Work out the finished part from the listing and answer in its coordinate system (mm). A direction names the side the tool comes from. Give positions to 0.01 mm unless a question says otherwise; leave off trailing zeros. Order: outer loops, then holes, each group sorted by start corner. A loop starts at its lowest first (then second) coordinate and runs counter-clockwise, first axis right, second up. Notation, with made-up numbers: (51.25, 36) - (76.25, 36) arc R27 ccw to (76.25, 61) - close; hole circle Ø10 at (7.5, 67.25). An arc over 180 degrees is marked (long way). Put each result on its own line as item: value.
```python
from build123d import *

# Parameters (mm, degrees)
CROQUIS2_W              = 51
CROQUIS2_H              = 50
SALIENTE_EXTRUIR3_DEPTH = 10
CROQUIS6_W              = 49
CROQUIS6_H              = 9
CORTAR_EXTRUIR4_DEPTH   = 50
CORTAR_EXTRUIR5_REACH   = 38.827
CROQUIS7_R              = 0.25
CORTAR_EXTRUIR7_REACH   = 38.827
CROQUIS10_R             = 0.25
CORTAR_EXTRUIR8_REACH   = 38.827
CROQUIS11_R             = 0.25
CORTAR_EXTRUIR9_REACH   = 38.827
CROQUIS12_R             = 0.25
CORTAR_EXTRUIR10_REACH  = 38.827
CROQUIS13_R             = 0.35


with BuildPart() as part:
    # Croquis2 → Saliente-Extruir3 (new body)
    with BuildSketch(Plane(origin=(0, 0, 0), x_dir=(1, 0, 0), z_dir=(0, 1, 0))):
        Rectangle(CROQUIS2_W, CROQUIS2_H)
    extrude(amount=SALIENTE_EXTRUIR3_DEPTH)

    # Croquis6 → Cortar-Extruir4 (cut)
    with BuildSketch(Plane.XY.offset(25)):
        with Locations((0, 5.5)):
            Rectangle(CROQUIS6_W, CROQUIS6_H)
    extrude(amount=-CORTAR_EXTRUIR4_DEPTH, mode=Mode.SUBTRACT)

    # Croquis7 → Cortar-Extruir5 (cut, up to next)
    with BuildSketch(Plane(origin=(0, 1, 0), x_dir=(1, 0, 0), z_dir=(0, 1, 0)), mode=Mode.PRIVATE) as cortar_extruir5_sk1:
        with Locations(Location((-20, 22.5, 0), (0, 0, 270))):
            Circle(CROQUIS7_R)
    cortar_extruir5_tool1 = extrude(cortar_extruir5_sk1.sketch, amount=-CORTAR_EXTRUIR5_REACH, mode=Mode.PRIVATE) & part.part
    add(cortar_extruir5_tool1.solids().sort_by_distance((-20, 1, -22.5))[0], mode=Mode.SUBTRACT)

    # Croquis10 → Cortar-Extruir7 (cut, up to next)
    with BuildSketch(Plane(origin=(0, 1, 0), x_dir=(1, 0, 0), z_dir=(0, 1, 0)), mode=Mode.PRIVATE) as cortar_extruir7_sk1:
        with Locations(Location((20, 22.5, 0), (0, 0, 270))):
            Circle(CROQUIS10_R)
    cortar_extruir7_tool1 = extrude(cortar_extruir7_sk1.sketch, amount=-CORTAR_EXTRUIR7_REACH, mode=Mode.PRIVATE) & part.part
    add(cortar_extruir7_tool1.solids().sort_by_distance((20, 1, -22.5))[0], mode=Mode.SUBTRACT)

    # Croquis11 → Cortar-Extruir8 (cut, up to next)
    with BuildSketch(Plane(origin=(0, 1, 0), x_dir=(1, 0, 0), z_dir=(0, 1, 0)), mode=Mode.PRIVATE) as cortar_extruir8_sk1:
        with Locations(Location((-20, -22.5, 0), (0, 0, 270))):
            Circle(CROQUIS11_R)
    cortar_extruir8_tool1 = extrude(cortar_extruir8_sk1.sketch, amount=-CORTAR_EXTRUIR8_REACH, mode=Mode.PRIVATE) & part.part
    add(cortar_extruir8_tool1.solids().sort_by_distance((-20, 1, 22.5))[0], mode=Mode.SUBTRACT)

    # Croquis12 → Cortar-Extruir9 (cut, up to next)
    with BuildSketch(Plane(origin=(0, 1, 0), x_dir=(1, 0, 0), z_dir=(0, 1, 0)), mode=Mode.PRIVATE) as cortar_extruir9_sk1:
        with Locations(Location((20, -22.5, 0), (0, 0, 270))):
            Circle(CROQUIS12_R)
    cortar_extruir9_tool1 = extrude(cortar_extruir9_sk1.sketch, amount=-CORTAR_EXTRUIR9_REACH, mode=Mode.PRIVATE) & part.part
    add(cortar_extruir9_tool1.solids().sort_by_distance((20, 1, 22.5))[0], mode=Mode.SUBTRACT)

    # Croquis13 → Cortar-Extruir10 (cut, up to next)
    with BuildSketch(Plane(origin=(0, 1, 0), x_dir=(1, 0, 0), z_dir=(0, 1, 0)), mode=Mode.PRIVATE) as cortar_extruir10_sk1:
        with Locations(Location((1.077350269, -16.5, 0), (0, 0, 270))):
            Circle(CROQUIS13_R)
    cortar_extruir10_tool1 = extrude(cortar_extruir10_sk1.sketch, amount=-CORTAR_EXTRUIR10_REACH, mode=Mode.PRIVATE) & part.part
    add(cortar_extruir10_tool1.solids().sort_by_distance((1.07735, 1, 16.5))[0], mode=Mode.SUBTRACT)


solid = part.part
```
(1) Section C-C, the plane x = -15 is taken. Write down the section's boundary in (y, z).
Geometry check:
outline: (0, -25) - (1, -25) - (1, 25) - (0, 25) - close
(2) Straight lines are drawn through the part: line 1 (Z direction, x = -20, y = 0.35); line 2 (X direction, y = 0.4, z = -22.5); line 3 (X direction, y = 9.75, z = 18). For each, find the intervals that lie inside material, in ascending order.
Geometry check:
line 1: z = -25 to -22.75, -22.25 to 22.25, 22.75 to 25
line 2: x = -25.5 to -20.25, -19.75 to 19.75, 20.25 to 25.5
line 3: x = -25.5 to -24.5, 24.5 to 25.5
(3) Section B-B, the plane z = -11 is taken. Write down the section's boundary in (x, y), then the cut area to 3 significant figures.
Geometry check:
outline: (-25.5, 0) - (25.5, 0) - (25.5, 10) - (24.5, 10) - (24.5, 1) - (-24.5, 1) - (-24.5, 10) - (-25.5, 10) - close
area: 69.0 mm²
(4) A tool of negligible diameter and unlimited length cuts with its end or side. For faces 4 (the face through (-25.5, 5, 0)), 5 (the face through (0, 1, 0)), from which of +Z, -Z, +X, -X, +Y, -Y can it reach the whole face along a straight path? Write none if from no direction.
Geometry check:
face 4: +Z, -Z, -X, +Y, -Y
face 5: +Z, -Z, +Y
(5) Determine the mould class of faces 1 (the face through (25.5, 5, 0)), 2 (the face through (-24.5, 5, 0)), 3 (the face through (-5.8, 0.2, 25)) for opening direction X: pulls with the +X half, pulls with the -X half, needs draft (parallel to the pull), parting line crosses it, or undercut.
Geometry check:
face 1: pulls with the +X half
face 2: undercut
face 3: needs draft
(6) Section A-A, the plane y = 7 is taken. Write down the section's boundary in (x, z), then the cut area to 3 significant figures.
Geometry check:
outline: (-25.5, -25) - (-24.5, -25) - (-24.5, 25) - (-25.5, 25) - close; (24.5, -25) - (25.5, -25) - (25.5, 25) - (24.5, 25) - close
area: 100 mm²
(7) Given pin 1 (1 mm diameter, centred on x = 0, z = -5, fed in from -Y), flat-ended and moving along its own axis, determine where the tip first touches the part or whether it passes through.
Geometry check:
pin 1: stops at y = 0
